from build123d import *

# Parameters (mm, degrees)
SKETCH1_W                = 19.05
SKETCH1_H                = 19.05
BOSS_EXTRUDE1_DEPTH      = 6.35
SKETCH2_W                = 19.05
SKETCH2_H                = 12.7
CUT_EXTRUDE1_DEPTH       = 5.08
SKETCH3_R                = 1.524
BOSS_EXTRUDE2_DEPTH      = 1.27
CHAMFER1_SIZE            = 1.27
CHAMFER1_OF_MIRROR1_SIZE = 1.27
SKETCH4_R                = 6.0325
BOSS_EXTRUDE3_DEPTH      = 12.7
FILLET1_R                = 5.08


with BuildPart() as part:
    # Sketch1 → Boss-Extrude1 (new, symmetric)
    with BuildSketch(Plane.XY):
        with Locations((9.525, -9.525)):
            Rectangle(SKETCH1_W, SKETCH1_H)
    extrude(amount=BOSS_EXTRUDE1_DEPTH, both=True)

    # Sketch2 → Cut-Extrude1 (cut, symmetric)
    with BuildSketch(Plane.XY):
        with Locations((9.525, -6.35)):
            Rectangle(SKETCH2_W, SKETCH2_H)
    extrude(amount=CUT_EXTRUDE1_DEPTH, both=True, mode=Mode.SUBTRACT)

    # Sketch3 → Boss-Extrude2 (add)
    with BuildSketch(Plane.XY.offset(-5.08)):
        with Locations((14.605, -6.096)):
            Circle(SKETCH3_R)
        with Locations((4.445, -6.096)):
            Circle(SKETCH3_R)
    boss_extrude2 = extrude(amount=BOSS_EXTRUDE2_DEPTH)

    # Chamfer1
    chamfer1_edges = [part.edges().sort_by_distance(p)[0] for p in [
        (13.081, -6.096, -3.81),
        (2.921, -6.096, -3.81),
    ]]
    chamfer(chamfer1_edges, length=CHAMFER1_SIZE - 0.0001)  # a hair under: the kernel refuses the full size

    # Mirror1: Boss-Extrude2 across plane
    add(boss_extrude2.mirror(Plane.XY))

    # Chamfer1 of Mirror1
    chamfer1_of_mirror1_edges = [part.edges().sort_by_distance(p)[0] for p in [
        (13.081, -6.096, 3.81),
        (2.921, -6.096, 3.81),
    ]]
    chamfer(chamfer1_of_mirror1_edges, length=CHAMFER1_OF_MIRROR1_SIZE - 0.0001)  # a hair under: the kernel refuses the full size

    # Sketch4 → Boss-Extrude3 (add)
    with BuildSketch(Plane.XZ.offset(19.05)):
        with Locations((9.525, 0)):
            Circle(SKETCH4_R)
    extrude(amount=BOSS_EXTRUDE3_DEPTH)

    # Fillet1
    fillet1_edges = [part.edges().sort_by_distance(p)[0] for p in [
        (3.4925, -31.75, 0),
    ]]
    fillet(fillet1_edges, radius=FILLET1_R)


solid = part.part
Read the model definition and answer for the solid it produces. Units are mm, in the model's axes. A direction names the side the tool comes from. Give positions to 0.01 mm unless a question says otherwise; leave off trailing zeros. Write each loop counter-clockwise with the first axis right and the second up, starting at its lowest first coordinate (ties: lowest second). Pieces come first, ordered by that corner, then holes. Notation, with made-up numbers: (46.25, 63) -> (67.25, 63) arc R23 cw to (67.25, 82) -> close; hole circle Ø10 at (-22, 46.25). An arc over 180 degrees is marked (long way). Answer as a JSON object with one key per item and string values. Group by question number.
1) A tool of negligible diameter and unlimited length cuts with its end or side. For faces 4 (the flat face through (9, 0, 6)), 5 (the cylindrical face through (3.5, -22.8, 0.3)), 6 (the conical face through (14.15, -6.08, 4.01)), from which of +Z, -Z, +X, -X, +Y, -Y can it reach the whole face along a straight path? Write none if from no direction.
2) Find section A-A (y = -10). Write down the section's boundary in (x, z).
3) The mould has two halves that part along X. Classify faces 1 (the flat face through (10, -31.75, 0)), 2 (the conical face through (4.386, -5.643, -4.013)), 3 (the flat face through (0, -14, 0)): +X half, -X half, draft (parallel to the pull), parting line (faces both ways), or undercut.
4) Each of these flat-tipped pins is pushed along its axis until it touches: P1, Ø1, axis at y = -21, z = -1.5, coming from the +X side; P2, Ø3, axis at y = -24.5, z = -5, coming from the +X side; P3, Ø3, axis at x = 6.5, z = -1.5, coming from the +Y side. Where does it stop, or does it pass through?
5) Find section B-B (y = -24.5). Write down the section's boundary in (x, z) (1 decimal).
6) Consider L1, parallel to Z at x = 10.75, y = -1.5; L2, parallel to Y at x = 3.75, z = -3.25; L3, parallel to Y at x = 9.5, z = -1. Determine where each line is inside the solid, lowest interval first. Write a range as from..to.
Values follow:
{
 "1": {"face 4": "+Z, -Z, +X, -X, +Y", "face 5": "-Y", "face 6": "none"},
 "2": {"outline": "(0, -6.35) -> (19.05, -6.35) -> (19.05, -5.08) -> (0, -5.08) -> close; (0, 5.08) -> (19.05, 5.08) -> (19.05, 6.35) -> (0, 6.35) -> close"},
 "3": {"face 1": "draft", "face 2": "undercut", "face 3": "-X half"},
 "4": {"P1": "stops at x = 15.47", "P2": "stops at x = 14.44", "P3": "stops at y = -12.7"},
 "5": {"outline": "circle Ø12.1 at (9.5, 0)"},
 "6": {"L1": "z = -6.35..-5.08, 5.08..6.35", "L2": "y = -19.05..-12.7", "L3": "y = -31.75..-12.7"}
}
